```python
from build123d import *

# Parameters (mm, degrees)
BOSS_EXTRUDE1_DEPTH = 6.35
SKETCH3_R           = 2.713000027
SKETCH3_R_2         = 2.663
CUT_EXTRUDE1_DEPTH  = 6.35


with BuildPart() as part:
    # Sketch1 → Boss-Extrude1 (new body)
    with BuildSketch(Plane(origin=(0, 0, 0), x_dir=(1, 0, 0), z_dir=(0, 1, 0))):
        Polygon((19.294897536, -16.615040594), (19.294897536, 79.223583745), (77.210897536, 79.223583745), (77.210897536, 142.723583745), (102.210897536, 142.723583745), (102.210897536, 79.223583745), (151.378897536, 79.223583745), (151.378897536, 142.723583745), (176.378897536, 142.723583745), (176.378897536, 79.223583745), (234.294897536, 79.223583745), (234.294897536, -16.615040594), (221.794897536, -16.615040594), (221.794897536, 66.777583745), (31.794897536, 66.777583745), (31.794897536, -16.615040594), align=None)
    extrude(amount=BOSS_EXTRUDE1_DEPTH)

    # Sketch3 → Cut-Extrude1 (cut)
    with BuildSketch(Plane.XZ):
        with Locations((84.779897535, -86.323583745)):
            Circle(SKETCH3_R)
        with Locations((94.649897535, -86.323583745)):
            Circle(SKETCH3_R_2)
        with Locations((84.779897535, -135.623583745)):
            Circle(SKETCH3_R_2)
        with Locations((94.649897535, -135.623583745)):
            Circle(SKETCH3_R_2)
        with Locations((158.939897536, -86.323583745)):
            Circle(SKETCH3_R_2)
        with Locations((168.809897536, -86.323583745)):
            Circle(SKETCH3_R_2)
        with Locations((158.939897536, -135.623583745)):
            Circle(SKETCH3_R_2)
        with Locations((168.809897536, -135.623583745)):
            Circle(SKETCH3_R_2)
    extrude(amount=-CUT_EXTRUDE1_DEPTH, mode=Mode.SUBTRACT)


solid = part.part
```
Read the model definition and answer for the solid it produces. Units are mm, in the model's axes. A direction names the side the tool comes from. Coordinates: 2 decimals unless noted, no trailing zeros. Write each loop counter-clockwise with the first axis right and the second up, starting at its lowest first coordinate (ties: lowest second). Pieces come first, ordered by that corner, then holes. Notation, with made-up numbers: (5.5, 6.5) -> (34.5, 6.5) arc R6 cw to (34.5, 13.5) -> close; hole circle Ø7 at (8, 49). An arc over 180 degrees is marked (long way). Answer as a JSON object with one key per item and string values.
Q1. Consider line 1 (X direction, y = 6, z = -112.5); line 2 (X direction, y = 5.75, z = -6); line 3 (Z direction, x = 194, y = 4.25). Determine where each line is inside the solid, lowest interval first. Write a range as [from, to].
The answers:
{"line 1": "x = [77.21, 102.21], [151.38, 176.38]", "line 2": "x = [19.29, 31.79], [221.79, 234.29]", "line 3": "z = [-79.22, -66.78]"}
Q2. Determine the mould class of faces 1 (the cylindrical face through (160.169, 3.131, -88.686)), 2 (the flat face through (164, 3, -142.724)), 3 (the cylindrical face through (96.082, 3.131, -133.378)), 4 (the flat face through (77.211, 3, -111)) for opening direction Z: pulls with the +Z half, pulls with the -Z half, needs draft (parallel to the pull), parting line crosses it, or undercut.
The answers:
{"face 1": "undercut", "face 2": "pulls with the -Z half", "face 3": "undercut", "face 4": "needs draft"}
Q3. The part is cut by section A-A on z = -125. Give the vertices of the cut face in (x, y), then the cut area to 4 significant figures.
The answers:
{"outline": "(77.21, 0) -> (102.21, 0) -> (102.21, 6.35) -> (77.21, 6.35) -> close; (151.38, 0) -> (176.38, 0) -> (176.38, 6.35) -> (151.38, 6.35) -> close", "area": "317.5 mm2"}
Q4. A tool of negligible diameter and unlimited length cuts with its end or side. For faces 5 (the flat face through (48, 3, -79.224)), 6 (the flat face through (102.211, 3, -111)), 7 (the flat face through (128, 3, -66.778)), from which of +Z, -Z, +X, -X, +Y, -Y can it reach the whole face along a straight path? Write none if from no direction.
The answers:
{"face 5": "-Z, -X, +Y, -Y", "face 6": "-Z, +Y, -Y", "face 7": "+Z, +Y, -Y"}
Q5. Flat-ended cylindrical pins translate along their axes: pin 1 Ø1 at (y, z) = (1.5, -83) entering from -X; pin 2 Ø4.5 at (x, z) = (158.94, -135.62) entering from +Y; pin 3 Ø1.9 at (x, y) = (198, 2) entering from -Z. Find the tip coordinate at first contact, or state that the pin passes through.
The answers:
{"pin 1": "stops at x = 77.21", "pin 2": "passes through", "pin 3": "stops at z = -79.22"}
Q6. The part is cut by section C-C on z = -54.5. Give the vertices of the cut face in (x, y).
The answers:
{"outline": "(19.29, 0) -> (31.79, 0) -> (31.79, 6.35) -> (19.29, 6.35) -> close; (221.79, 0) -> (234.29, 0) -> (234.29, 6.35) -> (221.79, 6.35) -> close"}
Q7. The part is cut by section D-D on x = 136.5. Give the vertices of the cut face in (y, z).
The answers:
{"outline": "(0, -79.22) -> (6.35, -79.22) -> (6.35, -66.78) -> (0, -66.78) -> close"}
Q8. The part is cut by section B-B on y = 2.25. Give the number of separate pieces and of enclosed holes in the cut face, then the cut area to 3 significant figures.
The answers:
{"separate pieces": "1", "enclosed holes": "8", "area": "7,760 mm2"}
